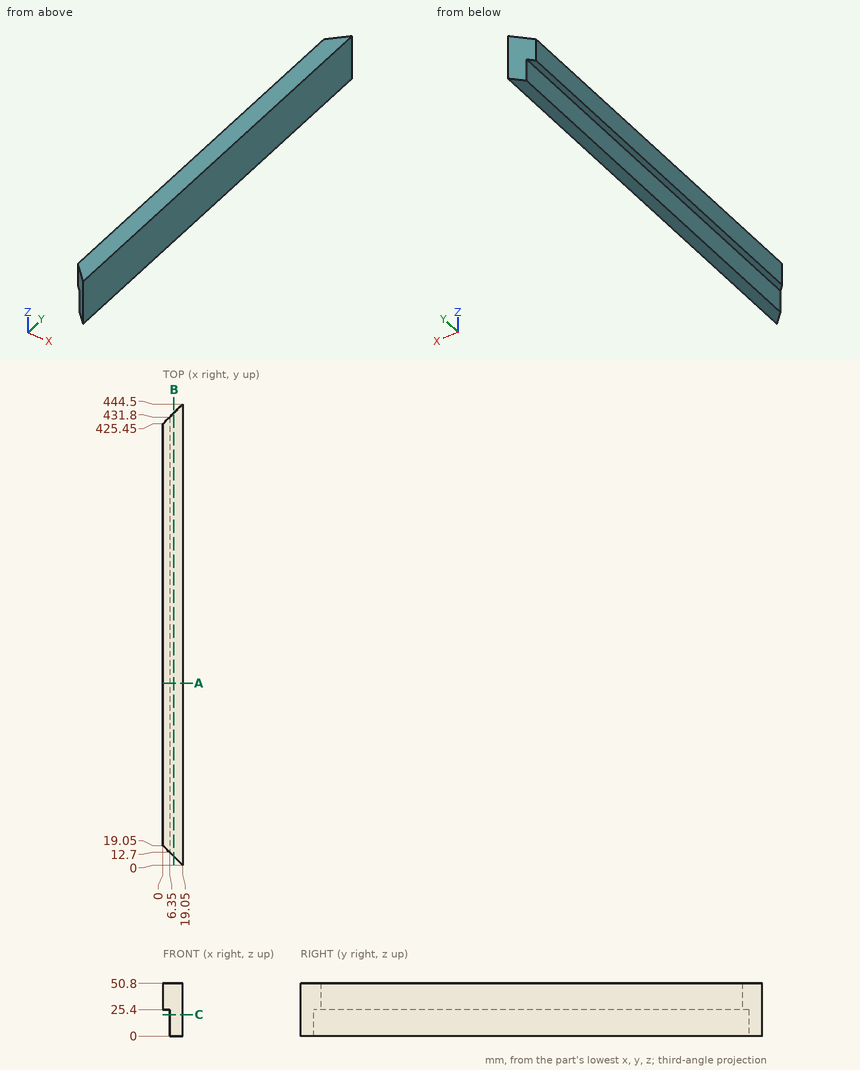
Job drawing, mm, ordinate dimensions from the low corner. One solid piece. Give positions to 0.01 mm unless a question says otherwise; leave off trailing zeros. Loops run counter-clockwise (first coordinate to the right, second up) from the corner with the lowest first, then second, coordinate; pieces in that order, holes last.
Item 1: Slice it at A-A, the plane y = 175.5. List the corners of the cut face in (x, z).
Answers follow:
outline: (0, 25.4) - (6.35, 25.4) - (6.35, 0) - (19.05, 0) - (19.05, 50.8) - (0, 50.8) - close
Item 2: Slice it at C-C, the plane z = 20.5. List the corners of the cut face in (x, y), and give its area (3 significant figures).
Answers follow:
outline: (6.35, 12.7) - (19.05, 0) - (19.05, 444.5) - (6.35, 431.8) - close
area: 5,480 mm2
Item 3: Flat gauge pins, fed straight in: pin 1 (3 mm diameter, centred on x = 12.5, z = 24.5, fed in from -Y); pin 2 (5 mm diameter, centred on x = 4, z = 9, fed in from -Y); pin 3 (3 mm diameter, centred on x = 6, z = 37, fed in from -Y). Where does each tip first touch, or does it go through?
Answers follow:
pin 1: stops at y = 5.05
pin 2: stops at y = 12.55
pin 3: stops at y = 11.55
Item 4: Slice it at B-B, the plane x = 10.5. List the corners of the cut face in (y, z).
Answers follow:
outline: (8.55, 0) - (435.95, 0) - (435.95, 50.8) - (8.55, 50.8) - close
Item 5: Drill centre lines: line 1 (X direction, y = 387.5, z = 10.5); line 2 (Z direction, x = 1, y = 220); line 3 (Y direction, x = 16, z = 16.5). Where is each one in solid material? Low to high.
Answers follow:
line 1: x = 6.35 to 19.05
line 2: z = 25.4 to 50.8
line 3: y = 3.05 to 441.45
